The listing builds one solid part. Answer for the finished solid, in the listing's coordinates (mm). A direction names the side the tool comes from. Coordinates: 2 decimals unless noted, no trailing zeros. Order: outer loops, then holes, each group sorted by start corner. A loop starts at its lowest first (then second) coordinate and runs counter-clockwise, first axis right, second up.
from build123d import *

# Parameters (mm, degrees)
SKETCH1_R           = 97.5
BOSS_EXTRUDE1_DEPTH = 650
SKETCH2_R           = 97.5
SKETCH2_R_2         = 67.5
CUT_EXTRUDE4_DEPTH  = 250
SKETCH4_R           = 67.5
CUT_EXTRUDE3_DEPTH  = 98.5
FILLET1_R           = 40


with BuildPart() as part:
    # Sketch1 → Boss-Extrude1 (new body)
    with BuildSketch(Plane(origin=(0, 0, 0), x_dir=(1, 0, 0), z_dir=(0, 1, 0))):
        Circle(SKETCH1_R)
    extrude(amount=BOSS_EXTRUDE1_DEPTH)

    # Sketch2 → Cut-Extrude4 (cut)
    with BuildSketch(Plane.XZ):
        Circle(SKETCH2_R)
        Circle(SKETCH2_R_2, mode=Mode.SUBTRACT)
    extrude(amount=-CUT_EXTRUDE4_DEPTH, mode=Mode.SUBTRACT)

    # Sketch4 → Cut-Extrude3 (cut, through all)
    with BuildSketch(Plane.XY):
        with Locations((0, 450)):
            Circle(SKETCH4_R)
    extrude(amount=-CUT_EXTRUDE3_DEPTH, mode=Mode.SUBTRACT)

    # Fillet1
    fillet1_edges = [part.edges().sort_by_distance(p)[0] for p in [
        (-97.5, 650, 0),
    ]]
    fillet(fillet1_edges, radius=FILLET1_R)


solid = part.part
(1) Find the intervals of material crossed by probe 1 along Y at (x, z) = (0, -36); probe 2 along Y at (x, z) = (0, -76); probe 3 along X at (y, z) = (450, -35), in increasing order.
(2) Find section B-B on y = 277.5. Determine the outline of the cut face in (x, z).
(3) A tool of negligible diameter and unlimited length cuts with its end or side. For faces 4 (the flat face through (-23, 250, -64)), 5 (the cylindrical face through (-21.14, 427.48, 95.18)), 6 (the cylindrical face through (-53.57, 408.93, -48.07)), from which of +Z, -Z, +X, -X, +Y, -Y can it reach the whole face along a straight path? Write none if from no direction.
(4) Find section D-D on y = 450. Determine the outline of the cut face in (x, z).
(5) Find section A-A on x = 0. Determine the outline of the cut face in (y, z).
(6) Find section C-C on y = 139. Determine the outline of the cut face in (x, z).
(7) Given pin 1 Ø10 at (x, y) = (50.5, 357) entering from +Z; pin 2 Ø5 at (x, y) = (-11.5, 321) entering from +Z; pin 3 Ø1 at (x, y) = (-43, 209.5) entering from +Z, each flat-ended and moving along its own axis, determine where each tip first touches the part or whether it passes through.
(8) The mould has two halves that part along X. Classify faces 1 (the flat face through (-1, 650, -1)), 2 (the flat face through (-1, 451, 0)), 3 (the cylindrical face through (-53.57, 123.25, -41.07)): pulls with the +X half, pulls with the -X half, needs draft (parallel to the pull), parting line crosses it, or undercut.
Resolved:
1. probe 1: y = 0 to 382.5, 517.5 to 650
1. probe 2: y = 250 to 382.5, 517.5 to 645.46
1. probe 3: x = -91 to -67.5, 67.5 to 91
2. outline: circle Ø195 at (0, 0)
3. face 4: -Y
3. face 5: +Y, -Y
3. face 6: -Z
4. outline: (-67.5, -70.36) - (-67.5, 0) - (67.5, 0) - (67.5, -70.36) arc R97.5 ccw (long way) to start
5. outline: (0, -67.5) - (250, -67.5) - (250, -97.5) - (382.5, -97.5) - (382.5, 0) - (517.5, 0) - (517.5, -97.5) - (610, -97.5) arc R40 ccw to (650, -57.5) - (650, 57.5) arc R40 ccw to (610, 97.5) - (250, 97.5) - (250, 67.5) - (0, 67.5) - close
6. outline: circle Ø135 at (0, 0)
7. pin 1: stops at z = 86.23
7. pin 2: stops at z = 97.08
7. pin 3: stops at z = 52.44
8. face 1: needs draft
8. face 2: undercut
8. face 3: parting line crosses it
